Could you check a few things on this drawing? It's one solid part, dimensions in mm from its lowest x, y, z. Coordinates: 2 decimals unless noted, no trailing zeros. Loops run counter-clockwise (first coordinate to the right, second up) from the corner with the lowest first, then second, coordinate; pieces in that order, holes last. Notation, with made-up numbers: (55, 37.5) -> (96, 37.5) arc R8 ccw to (96, 44.5) -> close; hole circle Ø11 at (86.5, -25). An arc over 180 degrees is marked (long way). One line per question, with ' | ' between items. Start each with the question number.
(1) I'm going to push flat-ended pins straight in: pin 1 Ø2.5 at (x, y) = (19.5, 1.5) entering from +Z; pin 2 Ø2.5 at (x, z) = (5.03, 33.32) entering from +Y; pin 3 Ø8 at (x, z) = (23, 15.5) entering from -Y; pin 4 Ø5 at (x, z) = (33.32, 5.03) entering from +Y. Where does each tip first touch, or does it pass through?
(2) If I drill on line 1 along Y through (x, z) = (27, 19.5); line 2 along Z through (x, y) = (14, 0.75); line 3 along Y through (x, z) = (13.5, 32), over which ranges is the centre line in solid material (lowest first)?
(3) Suppose I cut it at B-B (x = 34). Please give me the cut outline in (y, z), plus the area to 3 significant figures.
(4) Suppose I cut it at A-A (x = 14). Please give me the cut outline in (y, z).
(5) Suppose I cut it at C-C (z = 20). Please give me the cut outline in (x, y) (3 decimals).
(6) Suppose I cut it at D-D (y = 0.8). Please give me the cut outline in (x, z) (3 decimals), plus the area to 3 significant figures.
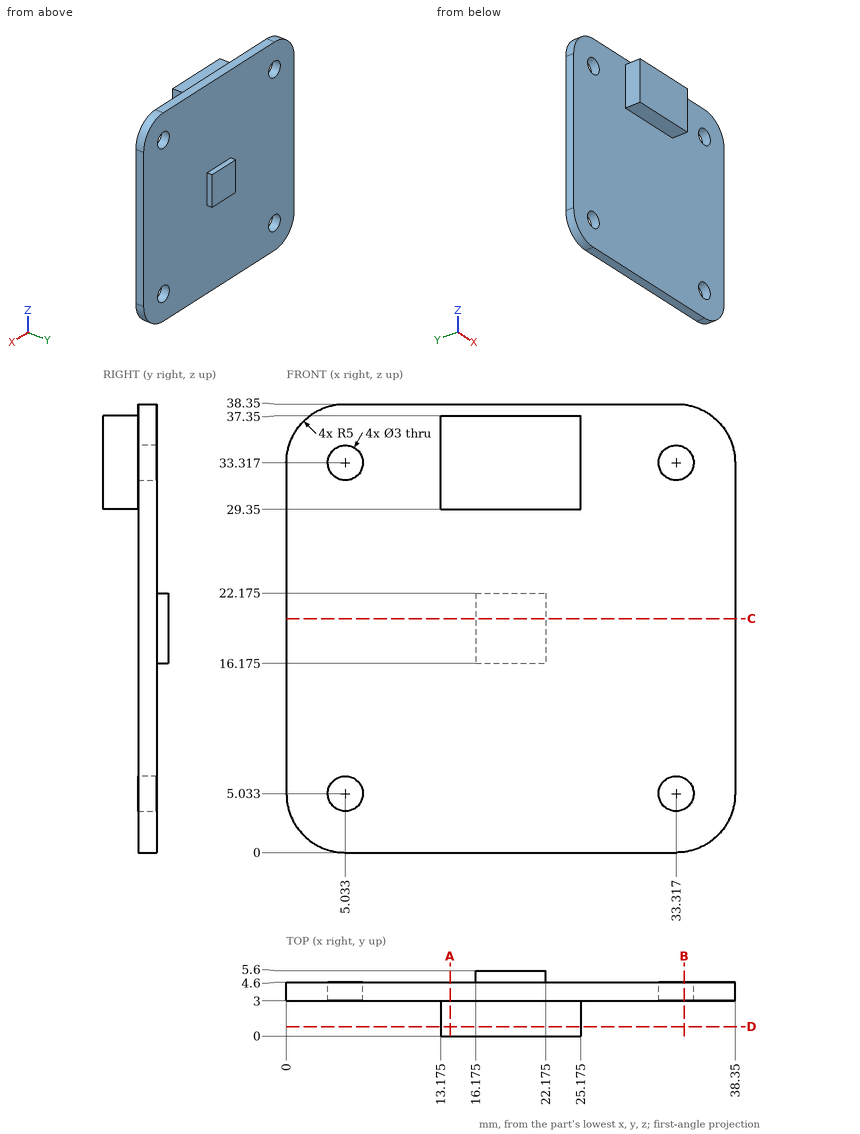
Checks:
1) pin 1: stops at z = 37.35 | pin 2: passes through | pin 3: stops at y = 3 | pin 4: stops at y = 4.6
2) line 1: y = 3 to 4.6 | line 2: z = 29.35 to 37.35 | line 3: y = 0 to 4.6
3) outline: (3, 0.04) -> (4.6, 0.04) -> (4.6, 3.7) -> (3, 3.7) -> close; (3, 6.37) -> (4.6, 6.37) -> (4.6, 31.98) -> (3, 31.98) -> close; (3, 34.65) -> (4.6, 34.65) -> (4.6, 38.31) -> (3, 38.31) -> close | area: 52.7 mm^2
4) outline: (0, 29.35) -> (3, 29.35) -> (3, 0) -> (4.6, 0) -> (4.6, 38.35) -> (3, 38.35) -> (3, 37.35) -> (0, 37.35) -> close
5) outline: (0, 3) -> (38.35, 3) -> (38.35, 4.6) -> (22.175, 4.6) -> (22.175, 5.6) -> (16.175, 5.6) -> (16.175, 4.6) -> (0, 4.6) -> close
6) outline: (13.175, 29.35) -> (25.175, 29.35) -> (25.175, 37.35) -> (13.175, 37.35) -> close | area: 96.0 mm^2
